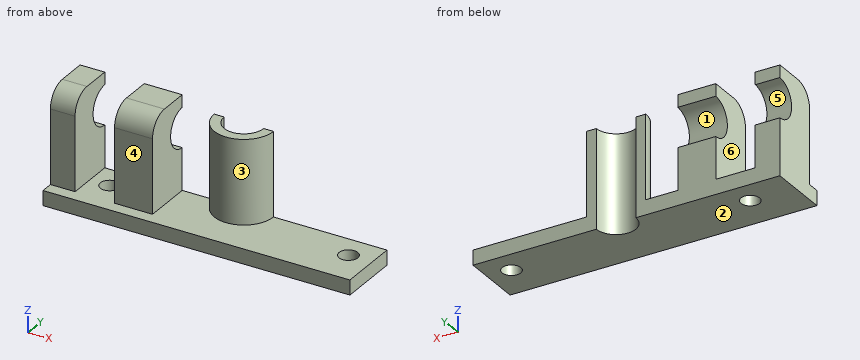
```python
from build123d import *

# Parameters (mm, degrees)
SKETCH1_W           = 58
SKETCH1_H           = 25
SKETCH1_R           = 1.9
BOSS_EXTRUDE1_DEPTH = 3
SKETCH2_R           = 6
BOSS_EXTRUDE2_DEPTH = 20
SKETCH3_R           = 4
CUT_EXTRUDE1_DEPTH  = 38.379807383
SKETCH4_W           = 7.7
SKETCH4_H           = 19.996282454
BOSS_EXTRUDE3_DEPTH = 19
CUT_EXTRUDE2_REACH  = 57.325
SKETCH5_R           = 4
FILLET1_R           = 4
SKETCH7_W           = 4.2
SKETCH7_H           = 25
BOSS_EXTRUDE4_DEPTH = 3
SKETCH8_W           = 5
SKETCH8_H           = 19.996282454
BOSS_EXTRUDE5_DEPTH = 19
CUT_EXTRUDE3_REACH  = 64.547
SKETCH9_R           = 4
FILLET2_R           = 4
SKETCH10_W          = 62.2
SKETCH10_H          = 12.5
CUT_EXTRUDE4_DEPTH  = 42.74314315


with BuildPart() as part:
    # Sketch1 → Boss-Extrude1 (new body)
    with BuildSketch(Plane.XY):
        Rectangle(SKETCH1_W, SKETCH1_H)
        with Locations((24.2, 5)):
            Circle(SKETCH1_R, mode=Mode.SUBTRACT)
        with Locations((24.2, -5)):
            Circle(SKETCH1_R, mode=Mode.SUBTRACT)
        with Locations((-24.2, 5)):
            Circle(SKETCH1_R, mode=Mode.SUBTRACT)
        with Locations((-24.2, -5)):
            Circle(SKETCH1_R, mode=Mode.SUBTRACT)
    extrude(amount=BOSS_EXTRUDE1_DEPTH)

    # Sketch2 → Boss-Extrude2 (add)
    with BuildSketch(Plane.XY):
        Circle(SKETCH2_R)
    extrude(amount=BOSS_EXTRUDE2_DEPTH)

    # Sketch3 → Cut-Extrude1 (cut, through all)
    with BuildSketch(Plane.XY.offset(20)):
        Circle(SKETCH3_R)
    extrude(amount=-CUT_EXTRUDE1_DEPTH, mode=Mode.SUBTRACT)

    # Sketch4 → Boss-Extrude3 (add)
    with BuildSketch(Plane.XY.offset(3)):
        with Locations((-16.35, 0)):
            Rectangle(SKETCH4_W, SKETCH4_H)
    extrude(amount=BOSS_EXTRUDE3_DEPTH)

    # Sketch5 → Cut-Extrude2 (cut, up to next)
    with BuildSketch(Plane.ZY.offset(20.2), mode=Mode.PRIVATE) as cut_extrude2_sk1:
        with Locations((15.5, 0.080826905)):
            Circle(SKETCH5_R)
    cut_extrude2_tool1 = extrude(cut_extrude2_sk1.sketch, amount=-CUT_EXTRUDE2_REACH, mode=Mode.PRIVATE) & part.part
    add(cut_extrude2_tool1.solids().sort_by_distance((-20.2, 0.080827, 15.5))[0], mode=Mode.SUBTRACT)

    # Fillet1
    fillet1_edges = [part.edges().sort_by_distance(p)[0] for p in [
        (-16.35, 9.998141227, 22),
        (-16.35, -9.998141227, 22),
    ]]
    fillet(fillet1_edges, radius=FILLET1_R)

    # Sketch7 → Boss-Extrude4 (add)
    with BuildSketch(Plane.XY.offset(3)):
        with Locations((-31.1, 0)):
            Rectangle(SKETCH7_W, SKETCH7_H)
    extrude(amount=-BOSS_EXTRUDE4_DEPTH)

    # Sketch8 → Boss-Extrude5 (add)
    with BuildSketch(Plane.XY.offset(3)):
        with Locations((-30.7, 0)):
            Rectangle(SKETCH8_W, SKETCH8_H)
    extrude(amount=BOSS_EXTRUDE5_DEPTH)

    # Sketch9 → Cut-Extrude3 (cut, up to next)
    with BuildSketch(Plane(origin=(-28.2, 0, 0), x_dir=(0, 0, -1), z_dir=(1, 0, 0)), mode=Mode.PRIVATE) as cut_extrude3_sk1:
        with Locations(Location((-15.5, 0.063578072, 0), (0, 0, 90))):
            Circle(SKETCH9_R)
    cut_extrude3_tool1 = extrude(cut_extrude3_sk1.sketch, amount=-CUT_EXTRUDE3_REACH, mode=Mode.PRIVATE) & part.part
    add(cut_extrude3_tool1.solids().sort_by_distance((-28.2, 0.063578, 15.5))[0], mode=Mode.SUBTRACT)

    # Fillet2
    fillet2_edges = [part.edges().sort_by_distance(p)[0] for p in [
        (-30.7, 9.998141227, 22),
        (-30.7, -9.998141227, 22),
    ]]
    fillet(fillet2_edges, radius=FILLET2_R)

    # Sketch10 → Cut-Extrude4 (cut, through all)
    with BuildSketch(Plane(origin=(0, 0, 0), x_dir=(-1, 0, 0), z_dir=(0, 0, -1))):
        with Locations((2.1, 6.25)):
            Rectangle(SKETCH10_W, SKETCH10_H)
    extrude(amount=-CUT_EXTRUDE4_DEPTH, mode=Mode.SUBTRACT)


solid = part.part
```
Verification items for the finished model (mm, model axes). Face numbers are marked on the shaded views. A direction names the side the tool comes from. Give positions to 0.01 mm unless a question says otherwise; leave off trailing zeros. Order: outer loops, then holes, each group sorted by start corner. A loop starts at its lowest first (then second) coordinate and runs counter-clockwise, first axis right, second up. Notation, with made-up numbers: M 24.25,-9.75 L 79.25,-9.75 A27 ccw 79.25,28.25 Z; hole C 72.25,35 d8. An arc over 180 degrees is marked long. Answer in a Markdown table with one row per item. Add a question column.
Item 1: Gauge pin test, flat ends, axial feed: pin 1 (3 mm diameter, centred on y = -7, z = 9.5, fed in from +X); pin 2 (6 mm diameter, centred on x = -5, y = -2.5, fed in from +Z); pin 3 (4 mm diameter, centred on y = -10.5, z = 8, fed in from +X). Record the tip position at first contact, or that the pin passes through.
Item 2: Section check D-D, the plane x = -17. Enter the section's corners in (y, z).
Item 3: Section check B-B, the plane x = -25. Enter the section's corners in (y, z), and give its area (3 significant figures).
Item 4: Scan lines: probe 1 along Y at (x, z) = (-24.2, 1); probe 2 along X at (y, z) = (-3, 20.25); probe 3 along Z at (x, y) = (6.5, -1.5). Record each from-to range of solid material in increasing order. Write a range as from..to.
Item 5: Section check A-A, the plane z = 9. Enter the section's corners in (x, y).
Item 6: Tool access check on the marked faces 4, 5 and 6. Record the directions out of +Z, -Z, +X, -X, +Y, -Y that give a thin tool (end or side, any length) a straight path to the whole face; none if there is none.
Item 7: Section check C-C, the plane y = -5. Enter the section's corners in (x, z).
Item 8: Mould release check, pull along Z, two halves, no side actions. Record for the marked faces 1, 2 and 3: released by +Z, released by -Z, zero draft, split by the parting line, or undercut.
Filled sheet:
| question | item | result |
|---|---|---|
| 1 | pin 1 | stops at x = 2.4 |
| 1 | pin 2 | stops at z = 20 |
| 1 | pin 3 | stops at x = -12.5 |
| 2 | outline | M -12.5,0 L 0,0 L 0,11.5 A4 cw 0,19.5 L 0,22 L -6,22 A4 ccw -10,18 L -10,3 L -12.5,3 Z |
| 3 | outline | M -12.5,0 L -6.72,0 L -6.72,3 L -12.5,3 Z; M -3.28,0 L 0,0 L 0,3 L -3.28,3 Z |
| 3 | area | 27.2 mm^2 |
| 4 | probe 1 | y = -12.5..-6.9, -3.1..0 |
| 4 | probe 2 | x = -33.2..-28.2, -20.2..-12.5 |
| 4 | probe 3 | z = 0..3 |
| 5 | outline | M -33.2,-10 L -28.2,-10 L -28.2,0 L -33.2,0 Z; M -20.2,-10 L -12.5,-10 L -12.5,0 L -20.2,0 Z; M -6,0 A6 ccw 6,0 L 4,0 A4 cw -4,0 Z |
| 6 | face 4 | +Z, +X, -X, -Y |
| 6 | face 5 | -X, +Y |
| 6 | face 6 | +Z, +Y, -Y |
| 7 | outline | M -33.2,0 L -26.1,0 L -26.1,3 L -28.2,3 L -28.2,22 L -33.2,22 Z; M -22.3,0 L 22.3,0 L 22.3,3 L 3.32,3 L 3.32,20 L -3.32,20 L -3.32,3 L -12.5,3 L -12.5,22 L -20.2,22 L -20.2,3 L -22.3,3 Z; M 26.1,0 L 29,0 L 29,3 L 26.1,3 Z |
| 8 | face 1 | undercut |
| 8 | face 2 | released by -Z |
| 8 | face 3 | zero draft |
